from build123d import *

# Parameters (mm, degrees)
SKETCH1_R           = 10
SKETCH1_R_2         = 5.15
BOSS_EXTRUDE1_DEPTH = 2
SKETCH3_R           = 3
BOSS_EXTRUDE2_DEPTH = 12
SKETCH4_R           = 10
SKETCH4_R_2         = 3
BOSS_EXTRUDE3_DEPTH = 2
CHAMFER2_SIZE       = 1
CHAMFER4_SIZE       = 0.5
CUT_EXTRUDE1_REACH  = 6
SKETCH5_R           = 0.75
SKETCH6_R           = 5.9
SKETCH6_R_2         = 5.15
BOSS_EXTRUDE4_DEPTH = 26
CUT_EXTRUDE2_REACH  = 32
SKETCH7_R           = 0.75


with BuildPart() as part:
    # Sketch1 → Boss-Extrude1 (new body)
    with BuildSketch(Plane.XY):
        Circle(SKETCH1_R)
        Circle(SKETCH1_R_2, mode=Mode.SUBTRACT)
    extrude(amount=BOSS_EXTRUDE1_DEPTH)



with BuildPart() as body_2:
    # Sketch3 → Boss-Extrude2 (new body)
    with BuildSketch(Plane(origin=(0, 0, 0), x_dir=(-1, 0, 0), z_dir=(0, 0, -1))):
        Circle(SKETCH3_R)
    extrude(amount=BOSS_EXTRUDE2_DEPTH)


with BuildPart() as part_1:
    add(part.part)

    add(body_2.part)  # Boss-Extrude3 merges body 2
    # Sketch4 → Boss-Extrude3 (add)
    with BuildSketch(Plane(origin=(0, 0, 0), x_dir=(-1, 0, 0), z_dir=(0, 0, -1))):
        Circle(SKETCH4_R)
        Circle(SKETCH4_R_2, mode=Mode.SUBTRACT)
    extrude(amount=BOSS_EXTRUDE3_DEPTH)

    # Chamfer2
    chamfer2_edges = [part_1.edges().sort_by_distance(p)[0] for p in [
        (3, 0, -2),
    ]]
    chamfer(chamfer2_edges, length=CHAMFER2_SIZE)

    # Chamfer4
    chamfer4_edges = [part_1.edges().sort_by_distance(p)[0] for p in [
        (3, 0, -12),
    ]]
    chamfer(chamfer4_edges, length=CHAMFER4_SIZE)

    # Sketch5 → Cut-Extrude1 (cut, up to next)
    with BuildSketch(Plane(origin=(0, 0, -2), x_dir=(-1, 0, 0), z_dir=(0, 0, -1)), mode=Mode.PRIVATE) as cut_extrude1_sk1:
        with Locations((-8.5, 0)):
            Circle(SKETCH5_R)
    cut_extrude1_tool1 = extrude(cut_extrude1_sk1.sketch, amount=-CUT_EXTRUDE1_REACH, mode=Mode.PRIVATE) & part_1.part
    add(cut_extrude1_tool1.solids().sort_by_distance((8.5, 0, -2))[0], mode=Mode.SUBTRACT)
    # Sketch5 → Cut-Extrude1 (cut, up to next)
    with BuildSketch(Plane(origin=(0, 0, -2), x_dir=(-1, 0, 0), z_dir=(0, 0, -1)), mode=Mode.PRIVATE) as cut_extrude1_sk2:
        with Locations((8.5, 0)):
            Circle(SKETCH5_R)
    cut_extrude1_tool2 = extrude(cut_extrude1_sk2.sketch, amount=-CUT_EXTRUDE1_REACH, mode=Mode.PRIVATE) & part_1.part
    add(cut_extrude1_tool2.solids().sort_by_distance((-8.5, 0, -2))[0], mode=Mode.SUBTRACT)

    # Sketch6 → Boss-Extrude4 (add)
    with BuildSketch(Plane.XY.offset(2)):
        Circle(SKETCH6_R)
        Circle(SKETCH6_R_2, mode=Mode.SUBTRACT)
    extrude(amount=BOSS_EXTRUDE4_DEPTH)

    # Sketch7 → Cut-Extrude2 (cut, up to next)
    with BuildSketch(Plane(origin=(0, 0, -2), x_dir=(-1, 0, 0), z_dir=(0, 0, -1)), mode=Mode.PRIVATE) as cut_extrude2_sk1:
        with Locations((0, 7.5)):
            Circle(SKETCH7_R)
    cut_extrude2_tool1 = extrude(cut_extrude2_sk1.sketch, amount=-CUT_EXTRUDE2_REACH, mode=Mode.PRIVATE) & part_1.part
    add(cut_extrude2_tool1.solids().sort_by_distance((0, 7.5, -2))[0], mode=Mode.SUBTRACT)
    # Sketch7 → Cut-Extrude2 (cut, up to next)
    with BuildSketch(Plane(origin=(0, 0, -2), x_dir=(-1, 0, 0), z_dir=(0, 0, -1)), mode=Mode.PRIVATE) as cut_extrude2_sk2:
        with Locations((6.495190528, -3.75)):
            Circle(SKETCH7_R)
    cut_extrude2_tool2 = extrude(cut_extrude2_sk2.sketch, amount=-CUT_EXTRUDE2_REACH, mode=Mode.PRIVATE) & part_1.part
    add(cut_extrude2_tool2.solids().sort_by_distance((-6.495191, -3.75, -2))[0], mode=Mode.SUBTRACT)
    # Sketch7 → Cut-Extrude2 (cut, up to next)
    with BuildSketch(Plane(origin=(0, 0, -2), x_dir=(-1, 0, 0), z_dir=(0, 0, -1)), mode=Mode.PRIVATE) as cut_extrude2_sk3:
        with Locations((-6.495190528, -3.75)):
            Circle(SKETCH7_R)
    cut_extrude2_tool3 = extrude(cut_extrude2_sk3.sketch, amount=-CUT_EXTRUDE2_REACH, mode=Mode.PRIVATE) & part_1.part
    add(cut_extrude2_tool3.solids().sort_by_distance((6.495191, -3.75, -2))[0], mode=Mode.SUBTRACT)


solid = part_1.part
Design review of the part built by this model. Coordinates are the model's own, in mm. A direction names the side the tool comes from. Round coordinates to 2 decimals unless told otherwise and drop trailing zeros. Write each loop counter-clockwise with the first axis right and the second up, starting at its lowest first coordinate (ties: lowest second). Pieces come first, ordered by that corner, then holes. Notation, with made-up numbers: M 68,67.5 L 102,67.5 A32 cw 102,94.5 Z; hole C 35.25,72.5 d10. An arc over 180 degrees is marked long. One line per item, written item: value. Start each with the question number.
1. Draft analysis for pull direction X (two halves, no side actions). For faces 1 (the face through (-7.75, 0.03, -0.03)), 2 (the face through (-4.3, 0.1, -2)), 3 (the face through (-5.894, 0.259, 14.818)), state which applies: pulls with the +X half, pulls with the -X half, needs draft (parallel to the pull), parting line crosses it, or undercut.
2. Take a section at B-B on y = 7.5. State the section outline as (x, z) points, then the cut area to 3 significant figures.
3. Take a section at A-A on x = 0. State the section outline as (y, z) points, then the cut area to 3 significant figures.
4. To check wall thickness, follow probe 1 along Y at (x, z) = (0, 1.55); probe 2 along Y at (x, z) = (-0.25, 10.5); probe 3 along Y at (x, z) = (8.5, 1.1). State the ranges of each line that lie inside material, in increasing order. Write a range as from..to.
5. Clearance check with flat-ended pins moving along their axes: P1, Ø1.7, axis at x = 8.5, y = 0, coming from the -Z side; P2, Ø4, axis at x = 2.5, z = 0.5, coming from the -Y side; P3, Ø1.8, axis at x = 0, y = 0.5, coming from the +Z side. State where each tip first meets the part, or that it passes through.
6. Take a section at C-C on z = 6.5. State the section outline as (x, y) points.
7. Take a section at D-D on x = -8.5. State the section outline as (y, z) points.
8. For faces 4 (the face through (-6.841, -4.415, -0.028)), 5 (the face through (4.3, -4.3, 2)), 6 (the face through (3, 0, -7)), list the 3-axis set-ups (+Z, -Z, +X, -X, +Y, -Y) from which the entire face can be reached by the end or side of a thin tool; tool diameter is ignored.
Computed:
1. face 1: undercut
1. face 2: needs draft
1. face 3: parting line crosses it
2. outline: M -6.61,-2 L -0.75,-2 L -0.75,2 L -6.61,2 Z; M 0.75,-2 L 6.61,-2 L 6.61,2 L 0.75,2 Z
2. area: 46.9 mm²
3. outline: M -10,-2 L -4,-2 L -3,-3 L -3,-11.5 L -2.5,-12 L 2.5,-12 L 3,-11.5 L 3,-3 L 4,-2 L 6.75,-2 L 6.75,2 L 5.9,2 L 5.9,28 L 5.15,28 L 5.15,0 L -5.15,0 L -5.15,28 L -5.9,28 L -5.9,2 L -10,2 Z; M 8.25,-2 L 10,-2 L 10,2 L 8.25,2 Z
3. area: 153 mm²
4. probe 1: y = -10..-5.15, 5.15..6.75, 8.25..10
4. probe 2: y = -5.89..-5.14, 5.14..5.89
4. probe 3: y = -5.27..-0.75, 0.75..5.27
5. P1: stops at z = -2
5. P2: stops at y = -9.99
5. P3: stops at z = 0
6. outline: C 0,0 d11.8; hole C 0,0 d10.3
7. outline: M -5.27,-2 L -0.75,-2 L -0.75,2 L -5.27,2 Z; M 0.75,-2 L 5.27,-2 L 5.27,2 L 0.75,2 Z
8. face 4: +Z, -Z
8. face 5: +Z
8. face 6: -Z
